from build123d import *

# Parameters (mm, degrees)
PAD_DEPTH       = 0.245
POCKET_DEPTH    = 0.05
SKETCH004_R     = 0.75
PAD001_DEPTH    = 10.08525
SKETCH005_R     = 3
HOLE_DEPTH      = 26
SKETCH006_R     = 0.495763
POCKET001_DEPTH = 9.580987


with BuildPart() as part:
    # Sketch → Pad (new body, symmetric)
    with BuildSketch(Plane.XY):
        with BuildLine():
            Line((0, 0.375), (19.21, 0.375))
            ThreePointArc((19.21, -0.375), (19.585, 0), (19.21, 0.375))
            Line((19.21, -0.375), (0, -0.375))
            ThreePointArc((0, 0.375), (-0.375, 0), (0, -0.375))
        make_face()
    extrude(amount=PAD_DEPTH, both=True)

    # Sketch001 → Revolution (revolve)
    with BuildSketch(Plane.XY):
        with BuildLine():
            Line((0, 0.625), (0, 0))
            Line((0, 0), (0, -0.625))
            ThreePointArc((0, 0.625), (-0.625, 0), (0, -0.625))
        make_face()
    revolve(axis=Axis((0, 0, 0), (0, -1, 0)))

    # Sketch002 → Revolution001 (revolve)
    with BuildSketch(Plane.XY):
        with BuildLine():
            ThreePointArc((19.21, -0.625), (19.835, 0), (19.21, 0.625))
            Line((19.21, 0.625), (19.21, 0))
            Line((19.21, 0), (19.21, -0.625))
        make_face()
    revolve(axis=Axis((19.21, 0, 0), (0, -1, 0)))

    # Sketch003 (on DatumPlane) → Pocket (cut)
    with BuildSketch(Plane.XY.offset(0.25)):
        Polygon((1.05425, -0.16238), (1.148, 0), (1.05425, 0.16238), (0.86675, 0.16238), (0.773, 0), (0.86675, -0.16238), align=None)
    extrude(amount=-POCKET_DEPTH, mode=Mode.SUBTRACT)

    # Sketch004 (on DatumPlane) → Pad001 (join)
    with BuildSketch(Plane.YZ.offset(11.526)):
        Circle(SKETCH004_R)
    extrude(amount=-PAD001_DEPTH)

    # Sketch005 (on DatumPlane) → Hole (cut)
    with BuildSketch(Plane.YZ.offset(11.526)):
        Circle(SKETCH005_R)
    extrude(amount=HOLE_DEPTH, mode=Mode.SUBTRACT)

    # Sketch006 (on DatumPlane) → Pocket001 (cut)
    with BuildSketch(Plane.YZ.offset(11.526)):
        Circle(SKETCH006_R)
    extrude(amount=-POCKET001_DEPTH, mode=Mode.SUBTRACT)


solid = part.part
Geometry check sheet. Reference: the model listing, model coordinates, mm. Round coordinates to 2 decimals unless told otherwise and drop trailing zeros. Loops run counter-clockwise (first coordinate to the right, second up) from the corner with the lowest first, then second, coordinate; pieces in that order, holes last. Notation, with made-up numbers: (36.5, 56) -> (51.5, 56) arc R22 cw to (51.5, 80) -> close; hole circle Ø1 at (-34.5, 5.5). An arc over 180 degrees is marked (long way). Answer as a JSON object with one key per item and string values. Group by question number.
Item 1: Release check for a two-part mould opening along Z. For faces 1 (the face through (6.803, -0.107, -0.484)), 2 (the face through (6.55, -0.75, 0.03)) record: pulls with the +Z half, pulls with the -Z half, needs draft (parallel to the pull), parting line crosses it, or undercut.
Item 2: Cross-section at A-A, the plane z = 0. Record the cut outline in (x, y) (3 decimals).
Item 3: Cross-section at B-B, the plane x = 9.25. Record the cut outline in (y, z).
Item 4: Depth check by flat-ended pin: pin 1 Ø0.5 at (x, z) = (1, 0) entering from -Y (3 decimals); pin 2 Ø0.6 at (x, y) = (1, 0) entering from +Z (3 decimals); pin 3 Ø0.6 at (x, y) = (1, 0) entering from -Z (3 decimals). Enter the tip coordinate at first touch or a pass-through.
Item 5: Thickness scan on line 1 along Z through (x, y) = (7.75, 0); line 2 along Y through (x, z) = (6.5, 0.05); line 3 along X through (y, z) = (-0.05, 0.55). Record the ranges inside material, lowest first.
Determined:
{
 "1": {"face 1": "undercut", "face 2": "parting line crosses it"},
 "2": {"outline": "(0.5, -0.375) -> (1.441, -0.375) -> (1.441, -0.75) -> (11.526, -0.75) -> (11.526, -0.496) -> (1.945, -0.496) -> (1.945, 0.496) -> (11.526, 0.496) -> (11.526, 0.75) -> (1.441, 0.75) -> (1.441, 0.375) -> (0.5, 0.375) arc R0.625 ccw (long way) to start"},
 "3": {"outline": "circle Ø1.5 at (0, 0); hole circle Ø0.99 at (0, 0)"},
 "4": {"pin 1": "stops at y = -0.375", "pin 2": "stops at z = 0.245", "pin 3": "stops at z = -0.245"},
 "5": {"line 1": "z = -0.75 to -0.5, 0.5 to 0.75", "line 2": "y = -0.75 to -0.49, 0.49 to 0.75", "line 3": "x = -0.29 to 0.29, 1.44 to 11.53"}
}
